Here's how the part is built. I have some questions about the finished solid (model axes, mm). Face numbers are marked on the shaded views. Round coordinates to 2 decimals unless told otherwise and drop trailing zeros. Loops run counter-clockwise (first coordinate to the right, second up) from the corner with the lowest first, then second, coordinate; pieces in that order, holes last. Notation, with made-up numbers: M 18.5,76 L 69.5,76 A12 cw 69.5,91 Z; hole C 9,66.5 d11. An arc over 180 degrees is marked long. Answer as a JSON object with one key per item and string values.
from build123d import *

# Parameters (mm, degrees)
F0_W     = 38.1
F0_H     = 38.1
F1_DEPTH = 19.05
F2_W     = 28.575
F2_H     = 28.575
F3_DEPTH = 6.35
F4_R     = 2.4892
F5_DEPTH = 25.4
F6_R     = 3.175
F7_DEPTH = 6.35
F8_SIZE  = 0.635


with BuildPart() as f1:
    # F0 (on Top) → F1 (new body)
    with BuildSketch(Plane.XY):
        with Locations((19.05, 19.05)):
            Rectangle(F0_W, F0_H)
    extrude(amount=F1_DEPTH)

    # F2 (on face) → F3 (cut)
    with BuildSketch(Plane.XY.offset(19.05)):
        with Locations((23.8125, 23.8125)):
            Rectangle(F2_W, F2_H)
    extrude(amount=-F3_DEPTH, mode=Mode.SUBTRACT)

    # F4 (on face) → F5 (cut)
    with BuildSketch(Plane.XY.offset(12.7)):
        with Locations((22.225, 22.225)):
            Circle(F4_R)
    extrude(amount=-F5_DEPTH, mode=Mode.SUBTRACT)

    # F6 (on face) → F7 (cut)
    with BuildSketch(Plane.XY.offset(19.05)):
        with Locations((9.525, 9.525)):
            Circle(F6_R)
    extrude(amount=-F7_DEPTH, mode=Mode.SUBTRACT)

    # F8
    f8_edges = [f1.edges().sort_by_distance(p)[0] for p in [
        (9.525, 25.4, 19.05),
        (7.279936, 7.279936, 19.05),
        (25.4, 9.525, 19.05),
        (38.1, 4.7625, 19.05),
        (19.05, 0, 19.05),
        (0, 19.05, 19.05),
        (4.7625, 38.1, 19.05),
        (0, 38.1, 9.525),
        (0, 0, 9.525),
        (0, 19.05, 0),
        (38.1, 0, 9.525),
        (19.05, 0, 0),
        (19.05, 38.1, 0),
        (38.1, 19.05, 0),
        (19.7358, 22.225, 0),
        (38.1, 38.1, 6.35),
        (38.1, 23.8125, 12.7),
        (38.1, 9.525, 15.875),
        (9.525, 38.1, 15.875),
        (23.8125, 38.1, 12.7),
        (19.7358, 22.225, 12.7),
    ]]
    chamfer(f8_edges, length=F8_SIZE)


solid = f1.part
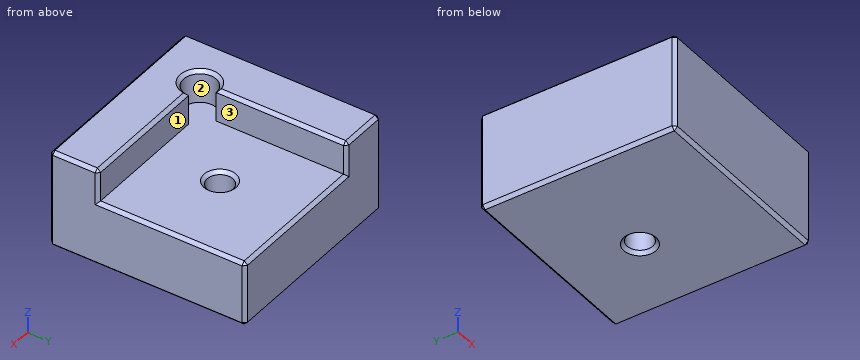
Item 1: If we mould it in two halves opening along X, with no side actions, what happens to the marked faces 1, 2 and 3? For each: pulls with the +X half, pulls with the -X half, needs draft (parallel to the pull), parting line crosses it, or undercut.
Resolved:
{"face 1": "needs draft", "face 2": "undercut", "face 3": "pulls with the +X half"}
Item 2: I want a section at A-A, the plane y = 17.5. Please give me the cut outline in (x, z) (3 decimals), then the cut area to 3 significant figures.
Resolved:
{"outline": "M 0,0.635 L 0.635,0 L 37.465,0 L 38.1,0.635 L 38.1,12.065 L 37.465,12.7 L 9.525,12.7 L 9.525,18.415 L 8.89,19.05 L 0.635,19.05 L 0,18.415 Z", "area": "543 mm²"}
Item 3: Please list where these lines run through material, in increasing order: probe 1 along Y at (x, z) = (22, 4.25); probe 2 along X at (y, z) = (30, 14.5) (3 decimals); probe 3 along Z at (x, y) = (25.5, 17.5). Write a range as from..to.
Resolved:
{"probe 1": "0..19.75, 24.7..38.1", "probe 2": "0..9.525", "probe 3": "0..12.7"}
Item 4: I'm going to push flat-ended pins straight in: pin 1 Ø6.5 at (x, z) = (19.5, 17) entering from +Y (3 decimals); pin 2 Ø2 at (x, y) = (21.5, 11) entering from +Z; pin 3 Ø3 at (x, y) = (22.225, 22.225) entering from +Z; pin 4 Ø3 at (y, z) = (19.5, 15) entering from +X (3 decimals). Where does each tip first touch, or does it pass through?
Resolved:
{"pin 1": "y = 9.525", "pin 2": "z = 12.7", "pin 3": "through", "pin 4": "x = 9.525"}
Item 5: I want a section at B-B, the plane z = 14. Please give me the cut outline in (x, y) (3 decimals).
Resolved:
{"outline": "M 0,0.635 L 0.635,0 L 37.465,0 L 38.1,0.635 L 38.1,8.89 L 37.465,9.525 L 12.7,9.525 A3.175 cw long 9.525,12.7 L 9.525,37.465 L 8.89,38.1 L 0.635,38.1 L 0,37.465 Z"}
